The listing builds one solid part. Answer for the finished solid, in the listing's coordinates (mm). Face numbers are marked on the shaded views. A direction names the side the tool comes from. Give positions to 0.01 mm unless a question says otherwise; leave off trailing zeros. Order: outer loops, then holes, each group sorted by start corner. A loop starts at its lowest first (then second) coordinate and runs counter-clockwise, first axis right, second up. Notation, with made-up numbers: (8.5, 20) - (45.5, 20) arc R30 cw to (45.5, 50) - close; hole circle Ø9 at (1.25, 59.25). An arc over 180 degrees is marked (long way). Answer in a Markdown table with one row per item.
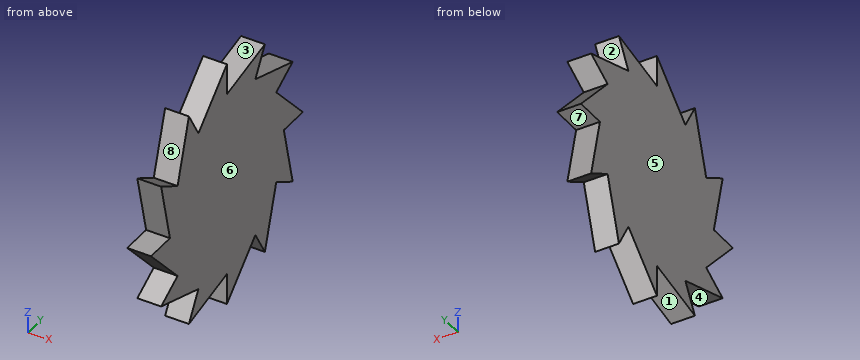
Autodesk Inventor part; units mm, degrees
ref_plane "XZ Plane" through (0, 0, 0) normal (0, 1, 0) x (-1, 0, 0)
ref_plane "XY Plane" through (0, 0, 0) normal (0, 0, 1) x (1, 0, 0)
sketch "Sketch1" plane through (0, 0, 0) normal (1, 0, 0) x (0, 1, 0)
  line L0 (16.4978, 9.525) -> (25.4, 0)
  line L1 (25.4, 0) -> (19.05, 0)
  line L2 (9.525, 16.4978) -> (21.997, 12.7)
  line L3 (21.997, 12.7) -> (16.4978, 9.525)
  line L4 (0, 19.05) -> (12.7, 21.997)
  line L5 (12.7, 21.997) -> (9.525, 16.4978)
  line L6 (-9.525, 16.4978) -> (0, 25.4)
  line L7 (0, 25.4) -> (0, 19.05)
  line L8 (-16.4978, 9.525) -> (-12.7, 21.997)
  line L9 (-12.7, 21.997) -> (-9.525, 16.4978)
  line L10 (-19.05, 0) -> (-21.997, 12.7)
  line L11 (-21.997, 12.7) -> (-16.4978, 9.525)
  line L12 (-16.4978, -9.525) -> (-25.4, 0)
  line L13 (-25.4, 0) -> (-19.05, 0)
  line L14 (-9.525, -16.4978) -> (-21.997, -12.7)
  line L15 (-21.997, -12.7) -> (-16.4978, -9.525)
  line L16 (0, -19.05) -> (-12.7, -21.997)
  line L17 (-12.7, -21.997) -> (-9.525, -16.4978)
  line L18 (9.525, -16.4978) -> (0, -25.4)
  line L19 (0, -25.4) -> (0, -19.05)
  line L20 (16.4978, -9.525) -> (12.7, -21.997)
  line L21 (12.7, -21.997) -> (9.525, -16.4978)
  line L22 (19.05, 0) -> (21.997, -12.7)
  line L23 (21.997, -12.7) -> (16.4978, -9.525)
  point P0 (0, 0)
  dimension "d7" = 360
ref_plane "Work Plane1" through (6.35, 0, 0) normal (1, 0, 0) x (0, 1, 0)
sketch "Sketch2" plane through (6.35, 0, 0) normal (1, 0, 0) x (0, 1, 0)
  line L0 (21.997, 12.7) -> (16.4978, 9.525)
  line L1 (16.4978, 9.525) -> (25.4, 0)
  line L2 (25.4, 0) -> (19.05, 0)
  line L3 (19.05, 0) -> (21.997, -12.7)
  line L4 (21.997, -12.7) -> (16.4978, -9.525)
  line L5 (16.4978, -9.525) -> (12.7, -21.997)
  line L6 (12.7, -21.997) -> (9.525, -16.4978)
  line L7 (9.525, -16.4978) -> (0, -25.4)
  line L8 (0, -25.4) -> (0, -19.05)
  line L9 (0, -19.05) -> (-12.7, -21.997)
  line L10 (-12.7, -21.997) -> (-9.525, -16.4978)
  line L11 (-9.525, -16.4978) -> (-21.997, -12.7)
  line L12 (-21.997, -12.7) -> (-16.4978, -9.525)
  line L13 (-16.4978, -9.525) -> (-25.4, 0)
  line L14 (-25.4, 0) -> (-19.05, 0)
  line L15 (-19.05, 0) -> (-21.997, 12.7)
  line L16 (-21.997, 12.7) -> (-16.4978, 9.525)
  line L17 (-16.4978, 9.525) -> (-12.7, 21.997)
  line L18 (-12.7, 21.997) -> (-9.525, 16.4978)
  line L19 (-9.525, 16.4978) -> (0, 25.4)
  line L20 (0, 25.4) -> (0, 19.05)
  line L21 (0, 19.05) -> (12.7, 21.997)
  line L22 (12.7, 21.997) -> (9.525, 16.4978)
  line L23 (9.525, 16.4978) -> (21.997, 12.7)
  point P0 (0, 0)
extrude "Extrusion1" add sketch "Sketch2" along normal blind 4.826
properties part number "ratchet_gear"
Item 1: Consider line 1 (Z direction, x = 9.8, y = 18); line 2 (Z direction, x = 8.95, y = -19); line 3 (Y direction, x = 7.4, z = -3). Determine where each line is inside the solid, lowest interval first.
Answer block:
| item | result |
|---|---|
| line 1 | -10.39 to 7.92, 10.39 to 13.92 |
| line 2 | -13.61 to -10.97, -6.85 to 10.97 |
| line 3 | -22.6 to 19.75 |
Item 2: Find section C-C on x = 9.15. Write down the section's boundary in (y, z) (3 decimals), then the cut area to 3 significant figures.
Answer block:
| item | result |
|---|---|
| outline | (-25.4, 0) - (-16.498, -9.525) - (-21.997, -12.7) - (-9.525, -16.498) - (-12.7, -21.997) - (0, -19.05) - (0, -25.4) - (9.525, -16.498) - (12.7, -21.997) - (16.498, -9.525) - (21.997, -12.7) - (19.05, 0) - (25.4, 0) - (16.498, 9.525) - (21.997, 12.7) - (9.525, 16.498) - (12.7, 21.997) - (0, 19.05) - (0, 25.4) - (-9.525, 16.498) - (-12.7, 21.997) - (-16.498, 9.525) - (-21.997, 12.7) - (-19.05, 0) - close |
| area | 1,450 mm² |
Item 3: Which of the six approach directions +Z, -Z, +X, -X, +Y, -Y give full straight-line access (tool end or side, diameter ignored) to the marked faces 1, 2, 3, 4 and 5?
Answer block:
| item | result |
|---|---|
| face 1 | -Z, +X, -X |
| face 2 | +X, -X, +Y |
| face 3 | +Z, +X, -X |
| face 4 | +X, -X, -Y |
| face 5 | +Z, -Z, -X, +Y, -Y |
Item 4: Find section A-A on y = -12. Write down the section's boundary in (x, z).
Answer block:
| item | result |
|---|---|
| outline | (6.35, -21.83) - (11.18, -21.83) - (11.18, -20.78) - (6.35, -20.78) - close; (6.35, -15.74) - (11.18, -15.74) - (11.18, 20.78) - (6.35, 20.78) - close |
Item 5: Find section B-B on z = -20. Write down the section's boundary in (x, y).
Answer block:
| item | result |
|---|---|
| outline | (6.35, -11.55) - (11.18, -11.55) - (11.18, -4.09) - (6.35, -4.09) - close; (6.35, 0) - (11.18, 0) - (11.18, 5.78) - (6.35, 5.78) - close; (6.35, 11.55) - (11.18, 11.55) - (11.18, 13.31) - (6.35, 13.31) - close |
Item 6: Each of these flat-tipped pins is pushed along its axis until it touches: P1, Ø2, axis at x = 9, y = -7.5, coming from the +Z side (3 decimals); P2, Ø1, axis at x = 10, y = 11, coming from the +Z side; P3, Ø1, axis at x = 9, y = 12.5, coming from the +Z side. Where does it stop, or does it pass through?
Answer block:
| item | result |
|---|---|
| P1 | z = 19.325 |
| P2 | z = 21.72 |
| P3 | z = 22 |
Item 7: Determine the mould class of the marked faces 6, 7 and 8 for opening direction Z: pulls with the +Z half, pulls with the -Z half, needs draft (parallel to the pull), parting line crosses it, or undercut.
Answer block:
| item | result |
|---|---|
| face 6 | needs draft |
| face 7 | undercut |
| face 8 | pulls with the +Z half |
